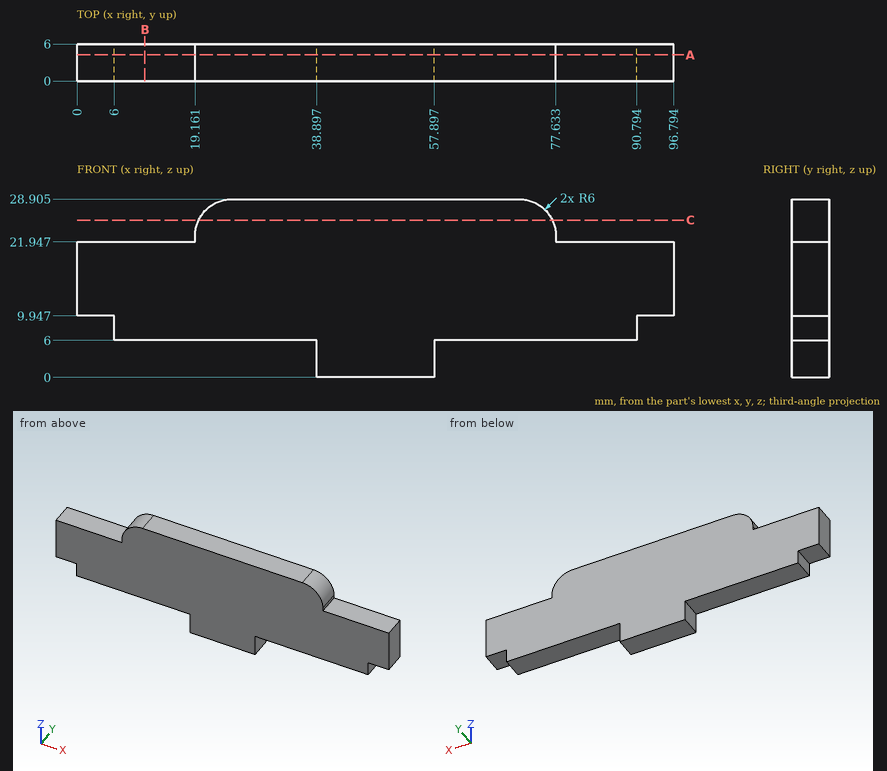
Geometry check sheet. Reference: drawing and pictorial views, mm from the part's lowest x, y, z. Give positions to 0.01 mm unless a question says otherwise; leave off trailing zeros. Order: outer loops, then holes, each group sorted by start corner. A loop starts at its lowest first (then second) coordinate and runs counter-clockwise, first axis right, second up. Notation, with made-up numbers: (81, 56.25) - (111, 56.25) arc R20 ccw to (111, 81.25) - close; hole circle Ø2 at (27.25, 49). An arc over 180 degrees is marked (long way). Answer as CSV lines item,"result". Start each with the question number.
Item 1: Gauge pin test, flat ends, axial feed: pin 1 (3 mm diameter, centred on y = 4, z = 7, fed in from -X); pin 2 (1.8 mm diameter, centred on x = 85, y = 2, fed in from +Z); pin 3 (3 mm diameter, centred on y = 3.5, z = 2, fed in from +X); pin 4 (2 mm diameter, centred on x = 32.5, z = 4.5, fed in from +Y). Record the tip position at first contact, or that the pin passes through.
Item 2: Section check A-A, the plane y = 4.25. Record the boundary of the cut face in (x, z) (1 decimal), plus the area to 3 significant figures.
Item 3: Material ranges on L1, parallel to Z at x = 29.5, y = 4.8 (1 decimal); L2, parallel to X at y = 4.3, z = 7 (1 decimal); L3, parallel to Z at x = 83, y = 2.6, recorded low to high.
Item 4: Section check C-C, the plane z = 25.5. Record the boundary of the cut face in (x, y), plus the area to 3 significant figures.
Item 5: Section check B-B, the plane x = 11. Record the boundary of the cut face in (y, z).
Filled in:
1,pin 1,"x = 6"
1,pin 2,"z = 21.95"
1,pin 3,"x = 57.9"
1,pin 4,"through"
2,outline,"(0, 9.9) - (6, 9.9) - (6, 6) - (38.9, 6) - (38.9, 0) - (57.9, 0) - (57.9, 6) - (90.8, 6) - (90.8, 9.9) - (96.8, 9.9) - (96.8, 21.9) - (77.6, 21.9) - (77.6, 22.9) arc R6 ccw to (71.6, 28.9) - (25.2, 28.9) arc R6 ccw to (19.2, 22.9) - (19.2, 21.9) - (0, 21.9) - close"
2,area,"2,000 mm^2"
3,L1,"6 to 28.9"
3,L2,"6 to 90.8"
3,L3,"6 to 21.95"
4,outline,"(19.75, 0) - (77.04, 0) - (77.04, 6) - (19.75, 6) - close"
4,area,"344 mm^2"
5,outline,"(0, 6) - (6, 6) - (6, 21.95) - (0, 21.95) - close"
